```python
from build123d import *

# Parameters (mm, degrees)
F0_W     = 20
F0_H     = 54
F1_DEPTH = 6.7
F3_DEPTH = 67.5
F4_R     = 2.550327
F4_R_2   = 2.5
F5_DEPTH = 25


with BuildPart() as f1:
    # F0 (on Front) → F1 (new body)
    with BuildSketch(Plane.XZ):
        with Locations((-25.59652, 16.161585)):
            Rectangle(F0_W, F0_H)
    extrude(amount=F1_DEPTH)

    # F2 (on face) → F3 (cut)
    with BuildSketch(Plane.XY.offset(43.161585)):
        Polygon((-20.79652, -1.810443), (-20.79652, 0), (-30.39652, 0), (-30.39652, -1.811175), (-33.09652, -1.811175), (-33.09652, -5.193342), (-18.09652, -5.193342), (-18.09652, -1.810443), align=None)
    extrude(amount=-F3_DEPTH, mode=Mode.SUBTRACT)

    # F4 (on face) → F5 (cut)
    with BuildSketch(Plane(origin=(0, -5.193342, 0), x_dir=(-1, 0, 0), z_dir=(0, 1, 0))):
        with Locations((26.046193, 19.544126)):
            Circle(F4_R)
        with Locations((26.09652, -3.912448)):
            Circle(F4_R_2)
    extrude(amount=-F5_DEPTH, mode=Mode.SUBTRACT)


solid = f1.part
```
The model under review builds one solid part; all positions refer to its coordinate system, in mm. A direction names the side the tool comes from. Give positions to 0.01 mm unless a question says otherwise; leave off trailing zeros. Write each loop counter-clockwise with the first axis right and the second up, starting at its lowest first coordinate (ties: lowest second). Pieces come first, ordered by that corner, then holes. Notation, with made-up numbers: M -2,-4.75 L 56,-4.75 A13 cw 56,4.25 Z; hole C 16,-14 d2. An arc over 180 degrees is marked long. Write item = value, one per line. Start each with the question number.
Q1. We need section C-C (z = 16). State the section outline as (x, y) points.
Q2. We need section A-A (y = -1.25). State the section outline as (x, z) points.
Q3. We need section D-D (x = -27.25). State the section outline as (y, z) points, plus the area to 3 significant figures.
Q4. Mouldability with a two-part tool opening along Z and no side actions: class faces 1 (the face through (-18.097, -4, 17)), 2 (the face through (-26, -6, -10.838)), 3 (the face through (-24.17, -5.94, 21.27)) as released by +Z, released by -Z, zero draft, split by the parting line, or undercut.
Q5. We need section B-B (x = -20.25). State the section outline as (y, z) points, plus the area to 3 significant figures.
Q6. Clearance check with a flat-ended pin moving along its axis: pin 1 (4 mm diameter, centred on x = -26.1, z = -3.91, fed in from -Y). State where the tip first meets the part, or that it passes through.
Q7. For line 1 (X direction, y = -0.5, z = 15); line 2 (X direction, y = -4.25, z = 20); line 3 (Y direction, x = -19, z = -8), list the stretches that pass through material, from the lowest coordinate up.
Q8. Machinability: for faces 4 (the face through (-33.097, -3, 17)), 5 (the face through (-20.797, -1, 17)), 6 (the face through (-15.597, -3, 16)), which of the approach directions +Z, -Z, +X, -X, +Y, -Y give a long, thin tool a straight path to every point of the face, cutting with its end or side? Answer none if there is none.
Result set:
q1.outline = M -35.6,-6.7 L -15.6,-6.7 L -15.6,0 L -20.8,0 L -20.8,-1.81 L -18.1,-1.81 L -18.1,-5.19 L -33.1,-5.19 L -33.1,-1.81 L -30.4,-1.81 L -30.4,0 L -35.6,0 Z
q2.outline = M -35.6,-10.84 L -30.4,-10.84 L -30.4,43.16 L -35.6,43.16 Z; M -20.8,-10.84 L -15.6,-10.84 L -15.6,43.16 L -20.8,43.16 Z
q3.outline = M -6.7,-10.84 L -5.19,-10.84 L -5.19,-6.13 L -6.7,-6.13 Z; M -6.7,-1.69 L -5.19,-1.69 L -5.19,17.3 L -6.7,17.3 Z; M -6.7,21.79 L -5.19,21.79 L -5.19,43.16 L -6.7,43.16 Z
q3.area = 67.9 mm2
q4.face_1 = zero draft
q4.face_2 = released by -Z
q4.face_3 = undercut
q5.outline = M -6.7,-10.84 L -5.19,-10.84 L -5.19,43.16 L -6.7,43.16 Z; M -1.81,-10.84 L 0,-10.84 L 0,43.16 L -1.81,43.16 Z
q5.area = 179 mm2
q6.pin_1 = through
q7.line_1 = -35.6 to -30.4, -20.8 to -15.6
q7.line_2 = -35.6 to -33.1, -18.1 to -15.6
q7.line_3 = -6.7 to -5.19, -1.81 to 0
q8.face_4 = +Z, -Z
q8.face_5 = +Z, -Z, +Y
q8.face_6 = +Z, -Z, +X, +Y, -Y
